The model under review builds one solid part; all positions refer to its coordinate system, in mm. Face numbers are marked on the shaded views. Coordinates: 2 decimals unless noted, no trailing zeros. Loops run counter-clockwise (first coordinate to the right, second up) from the corner with the lowest first, then second, coordinate; pieces in that order, holes last. Notation, with made-up numbers: M 43.5,39 L 54.5,39 A19 cw 54.5,62 Z; hole C 1.5,81 d3. An arc over 180 degrees is marked long. Write item = value, one per line. Start each with the question number.
Q1. We need section C-C on y = 6.5. Give the boundary of the cut face in (x, z) (3 decimals).
Q2. We need section A-A on y = -0.5. Count the separate pieces of the cut face and the enclosed holes in it, and give its area (3 significant figures).
Q3. Mouldability with a two-part tool opening along Z and no side actions: class the marked faces 1 and 2 as released by +Z, released by -Z, zero draft, split by the parting line, or undercut.
Q4. We need section B-B on z = 3.25. Give the boundary of the cut face in (x, y).
Q5. Clearance check with flat-ended pins moving along their axes: pin 1 Ø5 at (x, z) = (1, -1.5) entering from -Y; pin 2 Ø0.5 at (y, z) = (2.5, -7) entering from +X; pin 3 Ø2 at (x, y) = (-2, 3) entering from +Z. State where each tip first meets the part, or that it passes through.
Q6. Wall thickness on probe 1 along Z at (x, y) = (0, 2); probe 2 along Y at (x, z) = (0, -7.5); probe 3 along Z at (x, y) = (6, 4.25): over which ranges is each line inside the solid? List them lowest first.
Q7. We need section D-D on x = -4. Give the boundary of the cut face in (y, z).
from build123d import *

# Parameters (mm, degrees)
EXTRUDE_THIN1_DEPTH      = 8.5
EXTRUDE_THIN1_DEPTH_BACK = 8.5
SKETCH2_W                = 10
SKETCH2_H                = 2.5
SKETCH2_W_2              = 2.5
EXTRUDE1_DEPTH           = 10
EXTRUDE1_DEPTH_BACK      = 10
SKETCH3_W                = 6.25
SKETCH3_H                = 4
EXTRUDE2_DEPTH           = 10
SKETCH4_W                = 6.25
SKETCH4_H                = 4
EXTRUDE3_DEPTH           = 10


with BuildPart() as part:
    # Sketch1 → Extrude-Thin1 (new body, two sides)
    with BuildSketch(Plane(origin=(0, 0, 0), x_dir=(1, 0, 0), z_dir=(0, 1, 0))) as extrude_thin1_sk:
        with BuildLine():
            Line((7.523762622, -2.697363846), (5.345206482, -6.052046118))
            ThreePointArc((5.345206482, -6.052046118), (4.896883661, -6.537039014), (4.312382013, -6.844560207))
            Line((4.312382013, -6.844560207), (0.508155948, -8.080628184))
            ThreePointArc((0.508155948, -8.080628184), (0.194275162, -8.030914352), (0.05, -7.747758404))
            Line((0.05, -7.747758404), (0.05, -6.652305648))
            ThreePointArc((0.05, -6.652305648), (-0.006212483, -6.453404557), (-0.158219178, -6.313349383))
            ThreePointArc((-0.158219178, -6.313349383), (-0.35, -6.001152824), (-0.158219178, -5.688956264))
            ThreePointArc((-0.158219178, -5.688956264), (-0.006212483, -5.548901091), (0.05, -5.35))
            Line((0.05, -5.35), (0.05, 5.307179677))
            ThreePointArc((0.05, 5.307179677), (0.096891109, 5.482179677), (0.225, 5.610288568))
            ThreePointArc((0.225, 5.610288568), (0.45, 6), (0.225, 6.389711432))
            ThreePointArc((0.225, 6.389711432), (0.096891109, 6.517820323), (0.05, 6.692820323))
            Line((0.05, 6.692820323), (0.05, 7.751254615))
            ThreePointArc((0.05, 7.751254615), (-0.135496636, 8.115312262), (-0.539057647, 8.179230047))
            Line((-0.539057647, 8.179230047), (-4.343283713, 6.943162069))
            ThreePointArc((-4.343283713, 6.943162069), (-4.957759804, 6.619870559), (-5.429073538, 6.110006233))
            Line((-5.429073538, 6.110006233), (-7.607629679, 2.755323961))
            Line((-7.607629679, 2.755323961), (-7.523762622, 2.700860058))
            Line((-7.523762622, 2.700860058), (-5.345206482, 6.055542329))
            ThreePointArc((-5.345206482, 6.055542329), (-4.896883661, 6.540535225), (-4.312382013, 6.848056418))
            Line((-4.312382013, 6.848056418), (-0.508155948, 8.084124395))
            ThreePointArc((-0.508155948, 8.084124395), (-0.194275162, 8.034410563), (-0.05, 7.751254615))
            Line((-0.05, 7.751254615), (-0.05, 6.692820323))
            ThreePointArc((-0.05, 6.692820323), (0.010288568, 6.467820323), (0.175, 6.303108891))
            ThreePointArc((0.175, 6.303108891), (0.35, 6), (0.175, 5.696891109))
            ThreePointArc((0.175, 5.696891109), (0.010288568, 5.532179677), (-0.05, 5.307179677))
            Line((-0.05, 5.307179677), (-0.05, -5.35))
            ThreePointArc((-0.05, -5.35), (-0.091419724, -5.496558698), (-0.203424658, -5.599757248))
            ThreePointArc((-0.203424658, -5.599757248), (-0.45, -6.001152824), (-0.203424658, -6.4025484))
            ThreePointArc((-0.203424658, -6.4025484), (-0.091419724, -6.505746949), (-0.05, -6.652305648))
            Line((-0.05, -6.652305648), (-0.05, -7.747758404))
            ThreePointArc((-0.05, -7.747758404), (0.135496636, -8.111816051), (0.539057647, -8.175733836))
            Line((0.539057647, -8.175733836), (4.343283713, -6.939665858))
            ThreePointArc((4.343283713, -6.939665858), (4.957759804, -6.616374348), (5.429073538, -6.106510022))
            Line((5.429073538, -6.106510022), (7.607629679, -2.75182775))
            Line((7.607629679, -2.75182775), (7.523762622, -2.697363846))
        make_face()
    extrude(amount=EXTRUDE_THIN1_DEPTH)
    extrude(extrude_thin1_sk.sketch, amount=-EXTRUDE_THIN1_DEPTH_BACK)

    # Sketch2 → Extrude1 (cut, two sides)
    with BuildSketch(Plane(origin=(0, 0, 0), x_dir=(0, 0, -1), z_dir=(1, 0, 0))) as extrude1_sk:
        with Locations((0, 7.25)):
            Rectangle(SKETCH2_W, SKETCH2_H)
        with Locations((0, -7.25)):
            Rectangle(SKETCH2_W, SKETCH2_H)
        with Locations((8.25, 7.25)):
            Rectangle(SKETCH2_W_2, SKETCH2_H)
        with Locations((-8.25, 7.25)):
            Rectangle(SKETCH2_W_2, SKETCH2_H)
        with Locations((8.25, -7.25)):
            Rectangle(SKETCH2_W_2, SKETCH2_H)
        with Locations((-8.25, -7.25)):
            Rectangle(SKETCH2_W_2, SKETCH2_H)
    extrude(amount=EXTRUDE1_DEPTH, mode=Mode.SUBTRACT)
    extrude(extrude1_sk.sketch, amount=-EXTRUDE1_DEPTH_BACK, mode=Mode.SUBTRACT)

    # Sketch3 → Extrude2 (cut)
    with BuildSketch(Plane(origin=(0, 0, 0), x_dir=(-1, 0, 0), z_dir=(0, 0, 1))):
        with Locations((-3.225, -6.5)):
            Rectangle(SKETCH3_W, SKETCH3_H)
        with Locations((-3.225, 0)):
            Rectangle(SKETCH3_W, SKETCH3_H)
        with Locations((-3.225, 6.5)):
            Rectangle(SKETCH3_W, SKETCH3_H)
    extrude(amount=EXTRUDE2_DEPTH, mode=Mode.SUBTRACT)

    # Sketch4 → Extrude3 (cut)
    with BuildSketch(Plane(origin=(0, 0, 0), x_dir=(-1, 0, 0), z_dir=(0, 0, 1))):
        with Locations((3.225, 6.5)):
            Rectangle(SKETCH4_W, SKETCH4_H)
        with Locations((3.225, -0.062819576)):
            Rectangle(SKETCH4_W, SKETCH4_H)
        with Locations((3.225, -6.5)):
            Rectangle(SKETCH4_W, SKETCH4_H)
    extrude(amount=-EXTRUDE3_DEPTH, mode=Mode.SUBTRACT)


solid = part.part
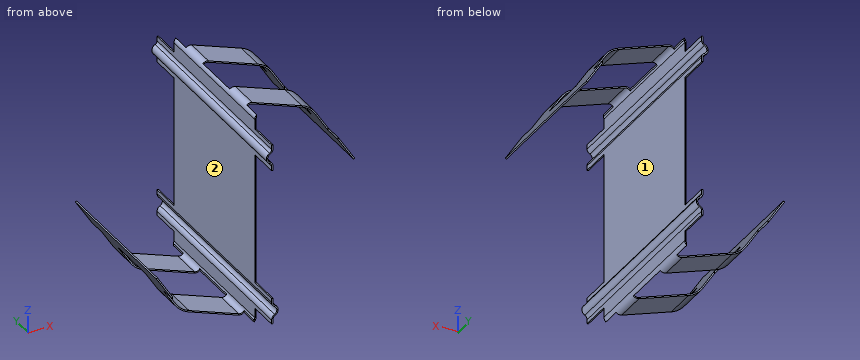
Returned:
q1.outline = M -0.203,5.6 A0.28 cw -0.05,5.35 L -0.05,5 L 0.05,5 L 0.05,5.35 A0.38 ccw -0.158,5.689 A0.35 cw -0.158,6.313 A0.38 ccw 0.05,6.652 L 0.05,7 L -0.05,7 L -0.05,6.652 A0.28 cw -0.203,6.403 A0.45 ccw Z; M -0.05,-7 L 0.05,-7 L 0.05,-6.693 A0.35 cw 0.225,-6.39 A0.45 ccw 0.225,-5.61 A0.35 cw 0.05,-5.307 L 0.05,-5 L -0.05,-5 L -0.05,-5.307 A0.45 ccw 0.175,-5.697 A0.35 cw 0.175,-6.303 A0.45 ccw -0.05,-6.693 Z
q2.separate_pieces = 3
q2.enclosed_holes = 0
q2.area = 2.11 mm^2
q3.face_1 = undercut
q3.face_2 = undercut
q4.outline = M -0.05,-6 L 0.05,-6 L 0.05,6 L -0.05,6 Z; M 7.16,-6 L 7.28,-6 L 7.28,6 L 7.16,6 Z
q5.pin_1 = -6
q5.pin_2 = 0.05
q5.pin_3 = -7.27
q6.probe_1 = -7.96 to -6.49, -5.51 to 5.54, 6.46 to 7.95
q6.probe_2 = -6 to 6
q6.probe_3 = 5.04 to 5.23
q7.outline = M -4.5,-7.05 L -1.94,-7.05 L -1.94,-6.95 L -4.5,-6.95 Z; M 2.06,-7.05 L 4.5,-7.05 L 4.5,-6.95 L 2.06,-6.95 Z
